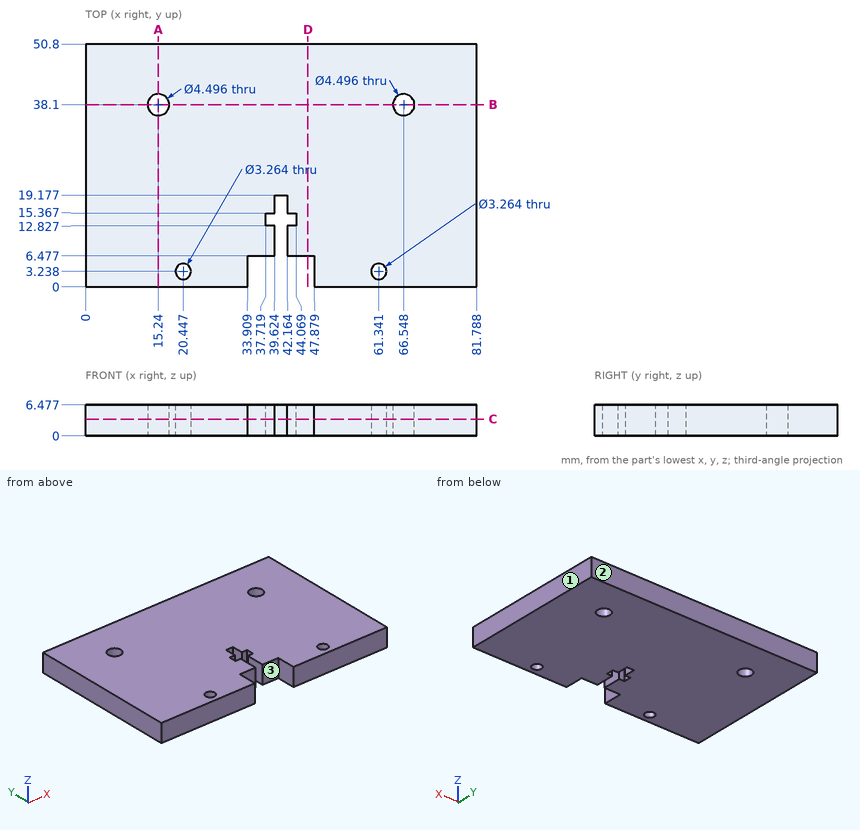
Source: three-view drawing plus pictorial views. Frame: mm from the lowest corner of the part. Give positions to 0.01 mm unless a question says otherwise; leave off trailing zeros. Write each loop counter-clockwise with the first axis right and the second up, starting at its lowest first coordinate (ties: lowest second). Pieces come first, ordered by that corner, then holes. Notation, with made-up numbers: (70.25, 81.25) - (114.25, 81.25) arc R34 cw to (114.25, 114.25) - close; hole circle Ø8 at (40.25, -27.5). An arc over 180 degrees is marked (long way). Write item = value, one per line. Start each with the question number.
Q1. Cut plane A-A, the plane x = 15.24. Return loops of the section in (y, z).
Q2. Pin query (flat end, axial travel): pin 1 Ø1.5 at (x, z) = (43.5, 4.5) entering from -Y; pin 2 Ø2 at (x, y) = (20.45, 3.24) entering from -Z. Return the tip coordinate at first contact, or that it passes through.
Q3. Cut plane C-C, the plane z = 3.5. Return loops of the section in (x, y) (1 decimal), then the cut area to 3 significant figures.
Q4. Draft query along X for the marked faces 1, 2 and 3. Return one class per face: +X half, -X half, draft (parallel to the pull), parting line (faces both ways), or undercut.
Q5. Cut plane B-B, the plane y = 38.1. Return loops of the section in (x, z) (1 decimal).
Q6. Cut plane D-D, the plane x = 46.5. Return loops of the section in (y, z).
Q7. Material intervals for probe 1 along Y at (x, z) = (15.24, 1.75); probe 2 along X at (y, z) = (15, 5); probe 3 along X at (y, z) = (16, 2) (1 decimal), sorted ascending.
Computed values:
q1.outline = (0, 0) - (35.85, 0) - (35.85, 6.48) - (0, 6.48) - close; (40.35, 0) - (50.8, 0) - (50.8, 6.48) - (40.35, 6.48) - close
q2.pin_1 = 6.48
q2.pin_2 = through
q3.outline = (0, 0) - (33.9, 0) - (33.9, 6.5) - (39.6, 6.5) - (39.6, 12.8) - (37.7, 12.8) - (37.7, 15.4) - (39.6, 15.4) - (39.6, 19.2) - (42.2, 19.2) - (42.2, 15.4) - (44.1, 15.4) - (44.1, 12.8) - (42.2, 12.8) - (42.2, 6.5) - (47.9, 6.5) - (47.9, 0) - (81.8, 0) - (81.8, 50.8) - (0, 50.8) - close; hole circle Ø4.5 at (15.2, 38.1); hole circle Ø3.3 at (20.4, 3.2); hole circle Ø3.3 at (61.3, 3.2); hole circle Ø4.5 at (66.5, 38.1)
q3.area = 3,970 mm²
q4.face_1 = +X half
q4.face_2 = draft
q4.face_3 = undercut
q5.outline = (0, 0) - (13, 0) - (13, 6.5) - (0, 6.5) - close; (17.5, 0) - (64.3, 0) - (64.3, 6.5) - (17.5, 6.5) - close; (68.8, 0) - (81.8, 0) - (81.8, 6.5) - (68.8, 6.5) - close
q6.outline = (6.48, 0) - (50.8, 0) - (50.8, 6.48) - (6.48, 6.48) - close
q7.probe_1 = 0 to 35.85, 40.35 to 50.8
q7.probe_2 = 0 to 37.72, 44.07 to 81.79
q7.probe_3 = 0 to 39.6, 42.2 to 81.8
